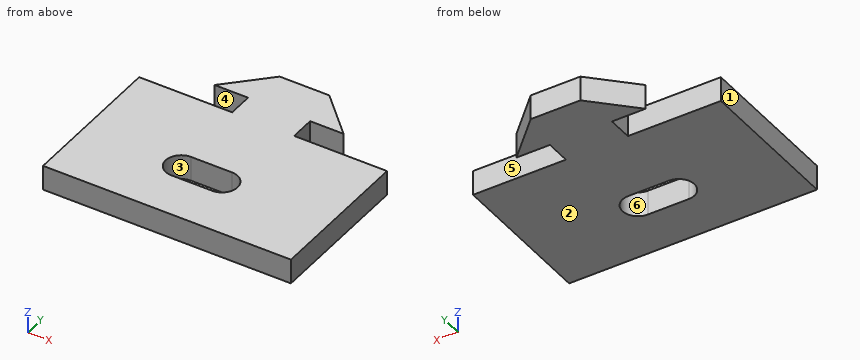
from build123d import *

# Parameters (mm, degrees)
PAD_DEPTH    = 2
POCKET_DEPTH = 5


with BuildPart() as part:
    # Sketch003 → Pad (new body)
    with BuildSketch(Plane.XY.offset(100)):
        Polygon((19.988775, -0.010854), (12.5, -0.010854), (12.5, 2), (15.2, 2), (12, 5.2), (8, 5.2), (4.8, 2), (7.5, 2), (7.5, 0), (0, 0), (0, -12.103219), (19.988775, -12.103219), align=None)
    extrude(amount=PAD_DEPTH)

    # Sketch (on Face13 of Pad) → Pocket (cut)
    with BuildSketch(Plane(origin=(0, 0, 100), x_dir=(1, 0, 0), z_dir=(0, 0, -1))):
        with BuildLine():
            ThreePointArc((7.917523, 8.322382), (6.665478, 7.070337), (7.917523, 5.818292))
            Line((7.917523, 5.818292), (11.208614, 5.818292))
            ThreePointArc((11.208614, 5.818292), (12.460659, 7.070337), (11.208614, 8.322382))
            Line((7.917523, 8.322382), (11.208614, 8.322382))
        make_face()
    extrude(amount=-POCKET_DEPTH, mode=Mode.SUBTRACT)


solid = part.part
Read the model definition and answer for the solid it produces. Units are mm, in the model's axes. Face numbers are marked on the shaded views. A direction names the side the tool comes from. Coordinates: 2 decimals unless noted, no trailing zeros. Write each loop counter-clockwise with the first axis right and the second up, starting at its lowest first coordinate (ties: lowest second). Pieces come first, ordered by that corner, then holes. Notation, with made-up numbers: M 30.5,80 L 51.5,80 A9 cw 51.5,93 Z; hole C -0.5,78.25 d4. An arc over 180 degrees is marked long. Use a Markdown table: item, result.
Q1. The part is cut by section A-A, the plane x = 10. Write down the section's boundary in (y, z), then the cut area to 3 significant figures.
Answer block:
| item | result |
|---|---|
| outline | M -12.1,100 L -8.32,100 L -8.32,102 L -12.1,102 Z; M -5.82,100 L 5.2,100 L 5.2,102 L -5.82,102 Z |
| area | 29.6 mm2 |
Q2. The part is cut by section C-C, the plane y = -6.5. Write down the section's boundary in (x, z), then the cut area to 3 significant figures.
Answer block:
| item | result |
|---|---|
| outline | M 0,100 L 6.8,100 L 6.8,102 L 0,102 Z; M 12.32,100 L 19.99,100 L 19.99,102 L 12.32,102 Z |
| area | 28.9 mm2 |
Q3. Determine the mould class of the marked faces 1, 2 and 3 for opening direction X: released by +X, released by -X, zero draft, split by the parting line, or undercut.
Answer block:
| item | result |
|---|---|
| face 1 | released by -X |
| face 2 | zero draft |
| face 3 | undercut |
Q4. Which of the six approach directions +Z, -Z, +X, -X, +Y, -Y give full straight-line access (tool end or side, diameter ignored) to the marked faces 4, 5 and 6?
Answer block:
| item | result |
|---|---|
| face 4 | +Z, -Z, -X |
| face 5 | +Z, -Z, +X |
| face 6 | +Z, -Z |
Q5. The part is cut by section D-D, the plane y = 3. Write down the section's boundary in (x, z), then the cut area to 3 significant figures.
Answer block:
| item | result |
|---|---|
| outline | M 5.8,100 L 14.2,100 L 14.2,102 L 5.8,102 Z |
| area | 16.8 mm2 |
Q6. Straight lines are drawn through the part: L1, parallel to Y at x = 1.25, z = 100.55; L2, parallel to X at y = -7.75, z = 100.9; L3, parallel to Y at x = 5.25, z = 100.7. For each, find the intervals that lie inside material, in ascending order. Write a range as [from, to].
Answer block:
| item | result |
|---|---|
| L1 | y = [-12.1, 0] |
| L2 | x = [0, 6.87], [12.26, 19.99] |
| L3 | y = [-12.1, 0], [2, 2.45] |
Q7. Each of these flat-tipped pins is pushed along its axis until it touches: pin 1 Ø4 at (x, y) = (5, 3) entering from -Z; pin 2 Ø1 at (y, z) = (1, 100.5) entering from +X; pin 3 Ø0.6 at (x, z) = (4, 101) entering from +Y. Where does it stop, or does it pass through?
Answer block:
| item | result |
|---|---|
| pin 1 | stops at z = 100 |
| pin 2 | stops at x = 12.5 |
| pin 3 | stops at y = 0 |
Q8. The part is cut by section B-B, the plane z = 101.45. Write down the section's boundary in (x, y).
Answer block:
| item | result |
|---|---|
| outline | M 0,-12.1 L 19.99,-12.1 L 19.99,-0.01 L 12.5,-0.01 L 12.5,2 L 15.2,2 L 12,5.2 L 8,5.2 L 4.8,2 L 7.5,2 L 7.5,0 L 0,0 Z; hole M 7.92,-8.32 L 11.21,-8.32 A1.25 ccw 11.21,-5.82 L 7.92,-5.82 A1.25 ccw Z |
